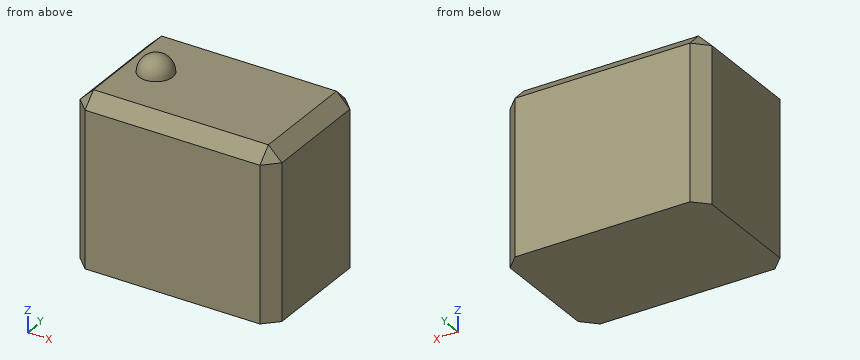
from build123d import *

# Parameters (mm, degrees)
F0_W     = 76.2
F0_H     = 50.8
F1_DEPTH = 63.5
F2_SIZE  = 5.08


with BuildPart() as f1:
    # F0 (on Top) → F1 (new body)
    with BuildSketch(Plane.XY):
        with Locations((6.05372, -4.891751)):
            Rectangle(F0_W, F0_H)
    extrude(amount=F1_DEPTH)

    # F2
    f2_edges = [f1.edges().sort_by_distance(p)[0] for p in [
        (-32.04628, 20.508249, 31.75),
        (6.05372, 20.508249, 63.5),
        (-32.04628, -4.891751, 63.5),
        (-32.04628, -30.291751, 31.75),
        (44.15372, -4.891751, 63.5),
        (44.15372, 20.508249, 31.75),
        (44.15372, -30.291751, 31.75),
        (6.05372, -30.291751, 63.5),
    ]]
    chamfer(f2_edges, length=F2_SIZE)

    # F3 (on face) → F4 (revolve)
    with BuildSketch(Plane.XY.offset(63.5)):
        with BuildLine():
            Line((-16.236074, -4.891751), (-16.236074, -11.241751))
            ThreePointArc((-16.236074, -11.241751), (-9.886074, -4.891751), (-16.236074, 1.458249))
            Line((-16.236074, 1.458249), (-16.236074, -4.891751))
        make_face()
    revolve(axis=Axis((-16.236074, -4.891751, 63.5), (0, -1, 0)))


solid = f1.part
Part model, mm, in its own coordinate system. Coordinates: 2 decimals unless noted, no trailing zeros. Order: outer loops, then holes, each group sorted by start corner. A loop starts at its lowest first (then second) coordinate and runs counter-clockwise, first axis right, second up.
(1) Probe L1, parallel to Z at x = -12.5, y = 12.5; L2, parallel to X at y = -5, z = 60; L3, parallel to X at y = -26, z = 23.5. List the from-to ranges inside material, lowest first.
Check sheet entries:
L1: z = 0 to 63.5
L2: x = -30.47 to 42.57
L3: x = -31.26 to 43.37
(2) Slice it at C-C, the plane z = 60.5. Write the cut outline in (x, y).
Check sheet entries:
outline: (-29.97, -25.21) - (-26.97, -28.21) - (39.07, -28.21) - (42.07, -25.21) - (42.07, 15.43) - (39.07, 18.43) - (-26.97, 18.43) - (-29.97, 15.43) - close
(3) Slice it at A-A, the plane y = 8. Write the cut outline in (x, z), and give its area (3 significant figures).
Check sheet entries:
outline: (-32.05, 0) - (44.15, 0) - (44.15, 58.42) - (39.07, 63.5) - (-26.97, 63.5) - (-32.05, 58.42) - close
area: 4,810 mm2
(4) Slice it at B-B, the plane x = 14.5. Write the cut outline in (y, z).
Check sheet entries:
outline: (-30.29, 0) - (20.51, 0) - (20.51, 58.42) - (15.43, 63.5) - (-25.21, 63.5) - (-30.29, 58.42) - close
(5) Pin check, flat tip, straight feed: pin 1 Ø4 at (x, y) = (-3, -19.5) entering from +Z. Stop position of the tip, or through.
Check sheet entries:
pin 1: stops at z = 63.5
